```python
from build123d import *

# Parameters (mm, degrees)
SKETCH1_W           = 99.3
SKETCH1_H           = 62.2
SKETCH1_R           = 2.275
SKETCH1_W_2         = 14
SKETCH1_H_2         = 14
BOSS_EXTRUDE1_DEPTH = 3
SKETCH6_W           = 99.3
SKETCH6_H           = 62.2
SKETCH6_R           = 1.5
SKETCH6_W_2         = 75.15
SKETCH6_H_2         = 18
BOSS_EXTRUDE2_DEPTH = 2
FILLET1_R           = 0.5


with BuildPart() as part:
    # Sketch1 → Boss-Extrude1 (new body)
    with BuildSketch(Plane(origin=(0, 0, 0), x_dir=(1, 0, 0), z_dir=(0, 1, 0))):
        with Locations((49.65, 31.1)):
            Rectangle(SKETCH1_W, SKETCH1_H)
        with Locations(Location((10, 37.2, 0), (0, 0, 270))):
            Circle(SKETCH1_R, mode=Mode.SUBTRACT)
        with Locations(Location((89.25, 52.2, 0), (0, 0, 270))):
            Circle(SKETCH1_R, mode=Mode.SUBTRACT)
        with Locations(Location((74.25, 25.05, 0), (0, 0, 270))):
            Circle(SKETCH1_R, mode=Mode.SUBTRACT)
        with Locations(Location((25, 15.05, 0), (0, 0, 270))):
            Circle(SKETCH1_R, mode=Mode.SUBTRACT)
        with Locations((11.525, 50.675)):
            Rectangle(SKETCH1_W_2, SKETCH1_H_2, mode=Mode.SUBTRACT)
        with Locations((30.575, 50.675)):
            Rectangle(SKETCH1_W_2, SKETCH1_H_2, mode=Mode.SUBTRACT)
        with Locations((49.625, 50.675)):
            Rectangle(SKETCH1_W_2, SKETCH1_H_2, mode=Mode.SUBTRACT)
        with Locations((68.675, 50.675)):
            Rectangle(SKETCH1_W_2, SKETCH1_H_2, mode=Mode.SUBTRACT)
        with Locations((87.725, 31.625)):
            Rectangle(SKETCH1_W_2, SKETCH1_H_2, mode=Mode.SUBTRACT)
        Polygon((75.675, 14.875), (84.35, 14.875), (84.35, 18.105), (91.1, 18.105), (91.1, 14.875), (91.925, 14.875), (91.925, 12.09), (91.1, 12.09), (91.1, 5.805), (89.375, 5.805), (89.375, 4.605), (86.075, 4.605), (86.075, 5.805), (84.35, 5.805), (84.35, 10.275), (75.675, 10.275), (75.675, 5.575), (61.675, 5.575), (61.675, 10.275), (53, 10.275), (53, 5.805), (51.275, 5.805), (51.275, 4.605), (47.975, 4.605), (47.975, 5.805), (46.25, 5.805), (46.25, 12.09), (45.425, 12.09), (45.425, 14.875), (46.25, 14.875), (46.25, 18.105), (53, 18.105), (53, 14.875), (61.675, 14.875), (61.675, 19.575), (75.675, 19.575), align=None, mode=Mode.SUBTRACT)
    extrude(amount=-BOSS_EXTRUDE1_DEPTH)

    # Sketch6 → Boss-Extrude2 (add)
    with BuildSketch(Plane.XZ.offset(3)):
        with Locations((49.65, -31.1)):
            Rectangle(SKETCH6_W, SKETCH6_H)
        with Locations(Location((89.25, -52.2, 0), (0, 0, 90))):
            Circle(SKETCH6_R, mode=Mode.SUBTRACT)
        with Locations(Location((74.25, -25.05, 0), (0, 0, 90))):
            Circle(SKETCH6_R, mode=Mode.SUBTRACT)
        with Locations(Location((25, -15.05, 0), (0, 0, 90))):
            Circle(SKETCH6_R, mode=Mode.SUBTRACT)
        with Locations(Location((10, -37.2, 0), (0, 0, 90))):
            Circle(SKETCH6_R, mode=Mode.SUBTRACT)
        Polygon((78.725, -21.575), (40.1, -21.575), (40.1, -1.575), (96.725, -1.575), (96.725, -40.625), (78.725, -40.625), align=None, mode=Mode.SUBTRACT)
        with Locations((40.1, -50.675)):
            Rectangle(SKETCH6_W_2, SKETCH6_H_2, mode=Mode.SUBTRACT)
    extrude(amount=BOSS_EXTRUDE2_DEPTH)

    # Fillet1
    fillet1_edges = [part.edges().sort_by_distance(p)[0] for p in [
        (49.65, 0, -62.2),
        (99.3, 0, -31.1),
        (49.65, 0, 0),
        (0, 0, -31.1),
        (0, -2.5, -62.2),
        (99.3, -2.5, -62.2),
        (99.3, -2.5, 0),
        (0, -2.5, 0),
    ]]
    fillet(fillet1_edges, radius=FILLET1_R)


solid = part.part
```
CAD build for the part. Positions are in the model's coordinates, mm. A direction names the side the tool comes from. Round coordinates to 2 decimals unless told otherwise and drop trailing zeros. Order: outer loops, then holes, each group sorted by start corner. A loop starts at its lowest first (then second) coordinate and runs counter-clockwise, first axis right, second up.
Q1. Which spindle directions (+Z, -Z, +X, -X, +Y, -Y) get a long thin tool onto all of the face, cutting with end or side? Do faces 4 (the flat face through (96.725, -4, -21)), 5 (the flat face through (88, -1, -4.605)), 6 (the flat face through (25, -3, -17)). Say none if no direction does.
Q2. Wall check: L1, parallel to X at y = -0.85, z = -25.05 (3 decimals); L2, parallel to X at y = -4.6, z = -52.2 (3 decimals); L3, parallel to Z at x = 46, y = -2.25 (3 decimals). Give the ranges that are in metal, low to high.
Q3. Slice it at D-D (z = -7). Write the cut outline in (x, y) (3 decimals).
Q4. Two-plate mould, pull along X, no slides. Class faces 1 (the flat face through (0, -3, -32)), 2 (the flat face through (40.1, -4, -12)), 3 (the flat face through (75.675, -1, -8)): pulls with the +X half, pulls with the -X half, needs draft (parallel to the pull), parting line crosses it, or undercut.
Q5. Slice it at B-B (z = -45). Write the cut outline in (x, y) (3 decimals), and give its area (3 significant figures).
Q6. Slice it at A-A (x = 10). Write the cut outline in (y, z) (3 decimals).
Q7. Slice it at C-C (x = 74.25). State how many separate pieces and enclosed holes the cut face has, and give its area (3 significant figures).
Q8. Drop a flat-ended pin along its axis: pin 1 (4 mm diameter, centred on x = 37.5, z = -54, fed in from -Y). Give the stop position or say it passes through.
Results below:
1. face 4: -Y
1. face 5: +Y, -Y
1. face 6: +Y
2. L1: x = 0 to 71.975, 76.525 to 80.725, 94.725 to 99.3
2. L2: x = 0 to 2.525, 77.675 to 87.75, 90.75 to 99.3
2. L3: z = -62.2 to -57.675, -43.675 to -14.875, -12.09 to 0
3. outline: (0, -5) - (40.1, -5) - (40.1, -3) - (46.25, -3) - (46.25, 0) - (0.5, 0) arc R0.5 ccw to (0, -0.5) - close; (53, -3) - (61.675, -3) - (61.675, 0) - (53, 0) - close; (75.675, -3) - (84.35, -3) - (84.35, 0) - (75.675, 0) - close; (91.1, -3) - (96.725, -3) - (96.725, -5) - (99.3, -5) - (99.3, -0.5) arc R0.5 ccw to (98.8, 0) - (91.1, 0) - close
4. face 1: pulls with the -X half
4. face 2: undercut
4. face 3: undercut
5. outline: (0, -5) - (2.525, -5) - (2.525, -3) - (4.525, -3) - (4.525, 0) - (0.5, 0) arc R0.5 ccw to (0, -0.5) - close; (18.525, -3) - (23.575, -3) - (23.575, 0) - (18.525, 0) - close; (37.575, -3) - (42.625, -3) - (42.625, 0) - (37.575, 0) - close; (56.625, -3) - (61.675, -3) - (61.675, 0) - (56.625, 0) - close; (75.675, -3) - (77.675, -3) - (77.675, -5) - (99.3, -5) - (99.3, -0.5) arc R0.5 ccw to (98.8, 0) - (75.675, 0) - close
5. area: 178 mm2
6. outline: (-5, -62.2) - (-0.5, -62.2) arc R0.5 ccw to (0, -61.7) - (0, -57.675) - (-3, -57.675) - (-3, -59.675) - (-5, -59.675) - close; (-5, -41.675) - (-3, -41.675) - (-3, -43.675) - (0, -43.675) - (0, -39.475) - (-3, -39.475) - (-3, -38.7) - (-5, -38.7) - close; (-5, -35.7) - (-3, -35.7) - (-3, -34.925) - (0, -34.925) - (0, -0.5) arc R0.5 ccw to (-0.5, 0) - (-5, 0) - close
7. separate pieces: 4
7. enclosed holes: 0
7. area: 131 mm2
8. pin 1: stops at y = -3
